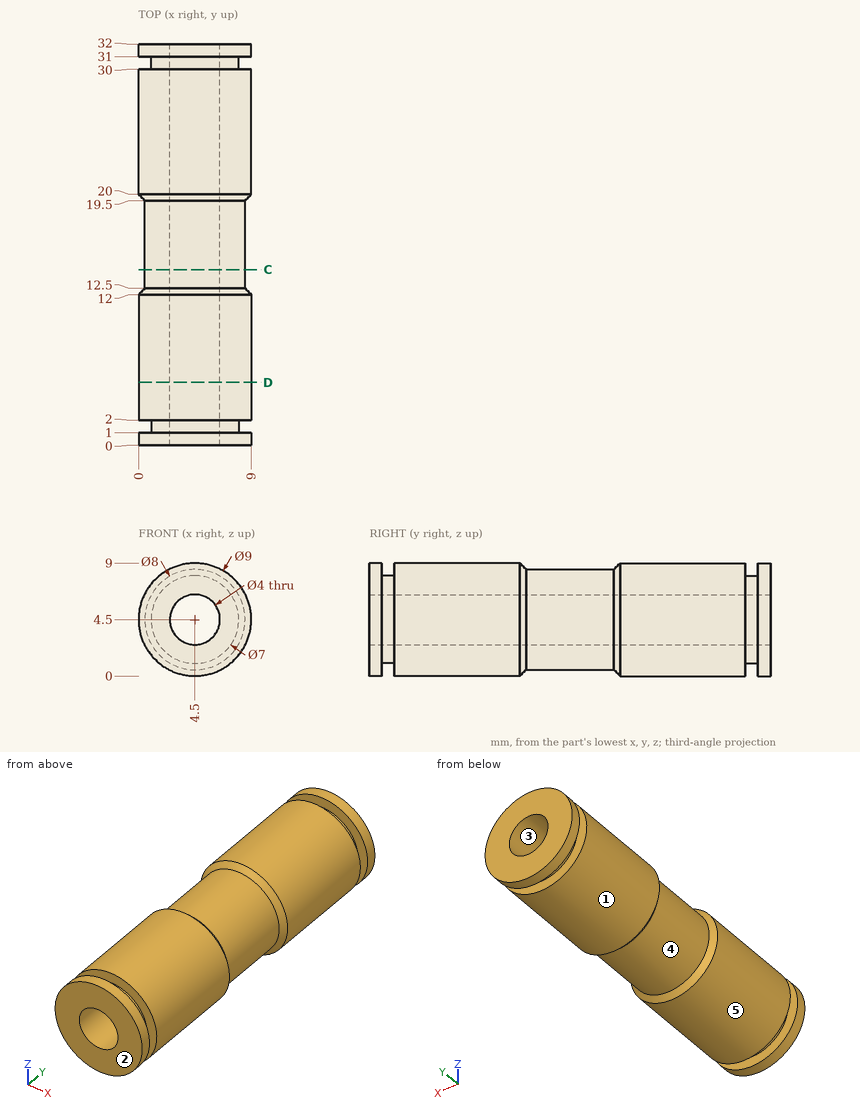
For this review, use the dimensioned drawing (mm, ordinates from the lowest corner) and the shaded views. A direction names the side the tool comes from. Round coordinates to 2 decimals unless told otherwise and drop trailing zeros. Write each loop counter-clockwise with the first axis right and the second up, starting at its lowest first coordinate (ties: lowest second). Pieces come first, ordered by that corner, then holes. Notation, with made-up numbers: (11, 77.5) - (16, 77.5) arc R30 ccw to (16, 104.5) - close; hole circle Ø5 at (-29.75, 36.5). An arc over 180 degrees is marked (long way). Answer as a JSON object with one key per item and string values.
1. We need section D-D on y = 5. Give the boundary of the cut face in (x, z), then the cut area to 3 significant figures.
Response values:
{"outline": "circle Ø9 at (4.5, 4.5); hole circle Ø4 at (4.5, 4.5)", "area": "51.1 mm2"}
2. To check wall thickness, follow line 1 along Y through (x, z) = (3.5, 1); line 2 along Z through (x, y) = (4.5, 18.5). State the ranges of each line that lie inside material, in increasing order.
Response values:
{"line 1": "y = 0 to 1, 2 to 30, 31 to 32", "line 2": "z = 0.5 to 2.5, 6.5 to 8.5"}
3. For pin 1 Ø1 at (y, z) = (12, 7.5) entering from +X; pin 2 Ø1 at (y, z) = (16, 4.5) entering from +X; pin 3 Ø2.5 at (x, z) = (4, 4.5) entering from +Y, all flat-tipped, find the tip position at first contact; note any pin that passes through.
Response values:
{"pin 1": "stops at x = 8.24", "pin 2": "stops at x = 8.5", "pin 3": "passes through"}
4. We need section C-C on y = 14. Give the boundary of the cut face in (x, z), then the cut area to 3 significant figures.
Response values:
{"outline": "circle Ø8 at (4.5, 4.5); hole circle Ø4 at (4.5, 4.5)", "area": "37.7 mm2"}
5. Draft analysis for pull direction X (two halves, no side actions). For the marked faces 1, 2 and 3, state which applies: +X half, -X half, draft (parallel to the pull), parting line (faces both ways), or undercut.
Response values:
{"face 1": "parting line", "face 2": "draft", "face 3": "undercut"}
6. Tool access review of the marked faces 4 and 5: name each direction out of +Z, -Z, +X, -X, +Y, -Y from which nothing blocks a thin tool from reaching the whole face with its end or side.
Response values:
{"face 4": "none", "face 5": "+Y, -Y"}
